```python
from build123d import *

# Parameters (mm, degrees)
F0_W      = 67.1
F0_H      = 138.3
F1_DEPTH  = 3.65
F2_R      = 5.08
F3_T      = -2.54
F4_W      = 19.863441
F4_H      = 9.705244
F5_DEPTH  = 12.5
F6_W      = 8.977096
F6_H      = 4.488549
F7_DEPTH  = 3
F8_W      = 3.636948
F8_H      = 9.400487
F8_W_2    = 3.415418
F8_H_2    = 16.339872
F9_DEPTH  = 8.3
F10_W     = 3.30219
F10_H     = 11.60476
F11_DEPTH = 4.7
F13_R     = 2.60328
F14_DEPTH = 4.1


with BuildPart() as f1:
    # F0 (on Front) → F1 (new body, symmetric)
    with BuildSketch(Plane.XZ):
        Rectangle(F0_W, F0_H)
    extrude(amount=F1_DEPTH, both=True)

    # F2
    f2_edges = [f1.edges().sort_by_distance(p)[0] for p in [
        (-33.55, 0, 69.15),
        (33.55, 0, 69.15),
        (33.55, 0, -69.15),
        (-33.55, 0, -69.15),
    ]]
    fillet(f2_edges, radius=F2_R)

    # F3
    f3_openings = [f1.faces().sort_by_distance(p)[0] for p in [
        (0, -3.65, 0),
    ]]
    offset(amount=F3_T, openings=f3_openings)

    # F4 (on face) → F5 (cut, symmetric)
    with BuildSketch(Plane(origin=(0, 3.65, 0), x_dir=(-1, 0, 0), z_dir=(0, 1, 0))):
        with Locations((-18.538279, 59.217378)):
            Rectangle(F4_W, F4_H)
    extrude(amount=F5_DEPTH, both=True, mode=Mode.SUBTRACT)

    # F6 (on face) → F7 (cut)
    with BuildSketch(Plane(origin=(0, 0, -69.15), x_dir=(1, 0, 0), z_dir=(0, 0, -1))):
        with Locations((-0.205018, 0.07035)):
            Rectangle(F6_W, F6_H)
    extrude(amount=-F7_DEPTH, mode=Mode.SUBTRACT)

    # F8 (on face) → F9 (cut, symmetric)
    with BuildSketch(Plane.YZ.offset(-31.01)):
        with Locations((-0.708474, 51.305823)):
            Rectangle(F8_W, F8_H)
        with Locations((-0.597709, 35.637243)):
            Rectangle(F8_W_2, F8_H_2)
    extrude(amount=F9_DEPTH, both=True, mode=Mode.SUBTRACT)

    # F10 (on face) → F11 (cut, symmetric)
    with BuildSketch(Plane(origin=(31.01, 0, 0), x_dir=(0, -1, 0), z_dir=(-1, 0, 0))):
        with Locations((0.541095, 43.273276)):
            Rectangle(F10_W, F10_H)
    extrude(amount=F11_DEPTH, both=True, mode=Mode.SUBTRACT)

    # F13 (on face) → F14 (cut, symmetric)
    with BuildSketch(Plane(origin=(0, 0, -69.15), x_dir=(1, 0, 0), z_dir=(0, 0, -1))):
        with Locations((-21.467019, 0)):
            Circle(F13_R)
    extrude(amount=F14_DEPTH, both=True, mode=Mode.SUBTRACT)


solid = f1.part
```
Here's how the part is built. I have some questions about the finished solid (model axes, mm). A direction names the side the tool comes from. Coordinates: 2 decimals unless noted, no trailing zeros. Write each loop counter-clockwise with the first axis right and the second up, starting at its lowest first coordinate (ties: lowest second). Pieces come first, ordered by that corner, then holes. Notation, with made-up numbers: M -29,81.5 L 20,81.5 A7 ccw 20,92.5 Z; hole C 81,-7 d8. An arc over 180 degrees is marked long. Answer as CSV lines item,"result". Start each with the question number.
Q1. Suppose I cut it at B-B, the plane z = 40.5. List the corners of the cut face in (x, y) for me.
Q2. Suppose I cut it at D-D, the plane y = 0. State how many separate pieces and enclosed holes the cut face has, then the cut area to 3 significant figures.
Q3. If we mould it in two halves opening along X, with no side actions, what happens to faces 5 (the flat face through (-32, -1, 46.606)), 6 (the flat face through (-33.55, 0, -1)), 7 (the cylindrical face through (-30.286, -1.237, 65.846))? For each: pulls with the +X half, pulls with the -X half, needs draft (parallel to the pull), parting line crosses it, or undercut.
Q4. For faces 1 (the flat face through (19, 2, 54.365)), 2 (the flat face through (32, -1, 49.076)), 3 (the flat face through (-4.694, 0, -68)), 4 (the cylindrical face through (30.286, -1.303, -65.846)), which set-ups out of +Z, -Z, +X, -X, +Y, -Y let a thin tool reach every point of the face, with its end or its side?
Q5. Will these pins go through, and if not, where does the flat tip stop? pin 1 Ø0.8 at (x, y) = (33, -1) entering from +Z; pin 2 Ø3 at (x, y) = (-32.5, -0.5) entering from -Z; pin 3 Ø1.3 at (x, y) = (-32.5, -1) entering from +Z.
Q6. Suppose I cut it at C-C, the plane x = -13.5. List the corners of the cut face in (y, z) for me, then the cut area to 3 significant figures.
Q7. I need wall thicknesses on probe 1 along Z at (x, y) = (13, -1.25); probe 2 along X at (y, z) = (0, -66.9); probe 3 along X at (y, z) = (-2.25, -19). Which ranges of each line are inside material? Lowest first, please. Write a range as [from, to].
Q8. Suppose I cut it at A-A, the plane x = 12.5. List the corners of the cut face in (y, z) for me.
Entries:
1,outline,"M -33.55,-3.65 L -31.01,-3.65 L -31.01,-2.31 L -33.55,-2.31 Z; M -33.55,1.11 L 33.55,1.11 L 33.55,3.65 L -33.55,3.65 Z; M 31.01,-3.65 L 33.55,-3.65 L 33.55,-2.19 L 31.01,-2.19 Z"
2,separate pieces,"5"
2,enclosed holes,"0"
2,area,"870 mm²"
3,face 5,"needs draft"
3,face 6,"pulls with the -X half"
3,face 7,"undercut"
4,face 1,"+Y, -Y"
4,face 2,"+X, -X"
4,face 3,"-Z"
4,face 4,"-Y"
5,pin 1,"stops at z = 67.03"
5,pin 2,"stops at z = -68.48"
5,pin 3,"stops at z = 67.86"
6,outline,"M -3.65,-69.15 L 3.65,-69.15 L 3.65,69.15 L -3.65,69.15 L -3.65,66.61 L 1.11,66.61 L 1.11,-66.61 L -3.65,-66.61 Z"
6,area,"375 mm²"
7,probe 1,"z = [-69.15, -66.61], [66.61, 69.15]"
7,probe 2,"x = [-32.69, -24.07], [-18.86, -4.69], [4.28, 32.69]"
7,probe 3,"x = [-33.55, -31.01], [31.01, 33.55]"
8,outline,"M -3.65,-69.15 L 3.65,-69.15 L 3.65,54.36 L 1.11,54.36 L 1.11,-66.61 L -3.65,-66.61 Z; M -3.65,66.61 L 1.11,66.61 L 1.11,64.07 L 3.65,64.07 L 3.65,69.15 L -3.65,69.15 Z"
